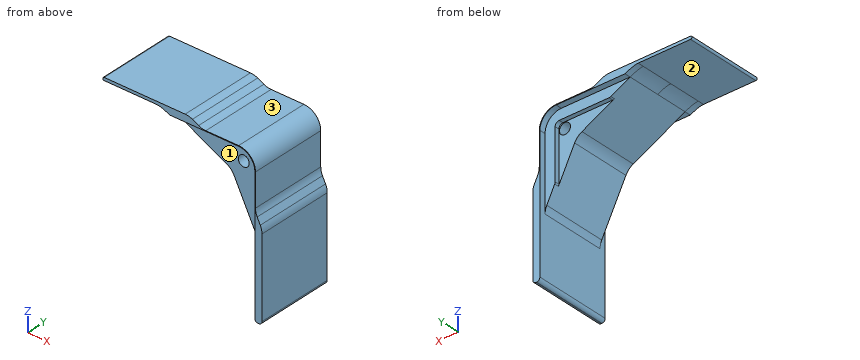
from build123d import *
from build123d.topology import SkipClean

# Parameters (mm, degrees)
SKETCH1_R           = 4.28625
BOSS_EXTRUDE1_DEPTH = 50.8
FILLET8_R           = 12.7
SKETCH2_W           = 42.1132
SKETCH2_H           = 3.302
CUT_EXTRUDE1_DEPTH  = 159.782890609
FILLET3_R           = 2.54
FILLET6_RADIUS      = 1.143
FILLET6_LENGTH      = 50.8
BOSS_EXTRUDE2_DEPTH = 30.1625
CUT_EXTRUDE2_DEPTH  = 163.081683202
FILLET7_R           = 12.7
SKETCH7_W           = 42.968170869
SKETCH7_H           = 42.968170869
CUT_EXTRUDE3_DEPTH  = 3.429
FILLET9_R           = 3.175


with BuildPart() as part:
    # Sketch1 → Boss-Extrude1 (new body)
    with BuildSketch(Plane(origin=(0, 0, 0), x_dir=(1, 0, 0), z_dir=(0, 1, 0))):
        with BuildLine():
            Line((12.7, 53.934971632), (-9.469611004, 9.469611004))
            Line((-9.469611004, 9.469611004), (-53.934971632, -12.7))
            Line((-53.934971632, -12.7), (-106.3752, -12.7))
            Line((-106.3752, -12.7), (-106.3752, -18.288))
            Line((-106.3752, -18.288), (0, -18.288))
            ThreePointArc((0, -18.288), (12.931568814, -12.931568814), (18.288, 0))
            Line((18.288, 0), (18.288, 106.3752))
            Line((18.288, 106.3752), (12.7, 106.3752))
            Line((12.7, 106.3752), (12.7, 53.934971632))
        make_face()
        with Locations(Location((0, 0, 0), (0, 0, 270))):
            Circle(SKETCH1_R, mode=Mode.SUBTRACT)
    extrude(amount=BOSS_EXTRUDE1_DEPTH)

    # Fillet8
    fillet8_edges = [part.edges().sort_by_distance(p)[0] for p in [
        (12.7, 25.4, -53.934971632),
        (-9.469611004, 25.4, -9.469611004),
    ]]
    fillet(fillet8_edges, radius=FILLET8_R)

    # Sketch2 → Cut-Extrude1 (cut, through all)
    with BuildSketch(Plane(origin=(0, 50.8, 0), x_dir=(1, 0, 0), z_dir=(0, 1, 0))):
        with Locations((-85.3186, -14.351)):
            Rectangle(SKETCH2_W, SKETCH2_H)
        with BuildLine():
            Line((-53.934971632, -12.7), (-64.262, -12.7))
            Line((-64.262, -12.7), (-64.262, -16.002))
            add(Edge.make_bspline(
                [(-53.934971632, -12.7), (-60.557759049, -16.002), (-64.262, -16.002)],
                knots=[0, 0, 0, 1, 1, 1], degree=2))
        make_face()
    extrude(amount=-CUT_EXTRUDE1_DEPTH, mode=Mode.SUBTRACT)

    # Fillet3
    fillet3_edges = [part.edges().sort_by_distance(p)[0] for p in [
        (12.7, 25.4, -106.3752),
        (18.288, 25.4, -106.3752),
    ]]
    fillet(fillet3_edges, radius=FILLET3_R)

    # Fillet6: full round fillet: the end face becomes a half cylinder, R = half its width
    fillet6_face = Plane((-106.3752, 25.4, 17.145), x_dir=(0, 1, 0), z_dir=(-1, 0, 0))  # on the end face: x along it, z out of the body
    fillet6_slab = fillet6_face.offset(-FILLET6_RADIUS / 2) * Box(FILLET6_LENGTH, 2 * FILLET6_RADIUS, FILLET6_RADIUS, mode=Mode.PRIVATE)  # the body's end, R deep
    fillet6_round = Plane((-105.2322, 25.4, 17.145), x_dir=(-1, 0, 0), z_dir=(0, 1, 0)) * Cylinder(FILLET6_RADIUS, FILLET6_LENGTH, mode=Mode.PRIVATE)  # its axis R under the face
    add(fillet6_slab - fillet6_round, mode=Mode.SUBTRACT)

    # Sketch3 → Boss-Extrude2 (add, symmetric)
    with SkipClean():  # the faces are left unmerged after this step: merging them gives an invalid solid
        with BuildSketch(Plane(origin=(0, 25.4, 0), x_dir=(1, 0, 0), z_dir=(0, 1, 0))):
            with BuildLine():
                Line((15.748, 106.3752), (15.24, 106.3752))
                ThreePointArc((15.24, 106.3752), (13.443948776, 105.631251224), (12.7, 103.8352))
                Line((12.7, 103.8352), (12.7, 0))
                ThreePointArc((12.7, 0), (8.980256121, -8.980256121), (0, -12.7))
                Line((0, -12.7), (-53.934971632, -12.7))
                add(Edge.make_bspline(
                    [(-53.934971632, -12.7), (-60.557759049, -16.002), (-64.262, -16.002)],
                    knots=[0, 0, 0, 1, 1, 1], degree=2))
                Line((-64.262, -16.002), (-105.2322, -16.002))
                ThreePointArc((-105.2322, -16.002), (-106.3752, -17.145), (-105.2322, -18.288))
                Line((-105.2322, -18.288), (0, -18.288))
                ThreePointArc((0, -18.288), (12.931568814, -12.931568814), (18.288, 0))
                Line((18.288, 0), (18.288, 103.8352))
                ThreePointArc((18.288, 103.8352), (17.544051224, 105.631251224), (15.748, 106.3752))
            make_face()
        extrude(amount=BOSS_EXTRUDE2_DEPTH, both=True)
    add(part.part.scale(1), mode=Mode.REPLACE)  # the faces are merged on a copy

    # Sketch6 → Cut-Extrude2 (cut, through all)
    with BuildSketch(Plane(origin=(0, 55.5625, 0), x_dir=(1, 0, 0), z_dir=(0, 1, 0))):
        with BuildLine():
            Line((-38.862, -18.288), (0, -18.288))
            ThreePointArc((0, -18.288), (12.931568814, -12.931568814), (18.288, 0))
            Line((18.288, 0), (18.288, 38.862))
            Line((18.288, 38.862), (13.208, 28.673096282))
            Line((13.208, 28.673096282), (13.208, 0))
            ThreePointArc((13.208, 0), (9.339466366, -9.339466366), (0, -13.208))
            Line((0, -13.208), (-28.673096282, -13.208))
            Line((-28.673096282, -13.208), (-38.862, -18.288))
        make_face()
    extrude(amount=-CUT_EXTRUDE2_DEPTH, mode=Mode.SUBTRACT)

    # Fillet7
    fillet7_edges = [part.edges().sort_by_distance(p)[0] for p in [
        (13.208, 25.4, -28.673096282),
        (18.288, 25.4, -38.862),
        (-38.862, 25.4, 18.288),
        (-28.673096282, 25.4, 13.208),
    ]]
    fillet(fillet7_edges, radius=FILLET7_R)

    # Sketch7 → Cut-Extrude3 (cut)
    with BuildSketch(Plane(origin=(0, 50.8, 0), x_dir=(1, 0, 0), z_dir=(0, 1, 0))):
        with Locations((-16.658085435, 16.658085435)):
            Rectangle(SKETCH7_W, SKETCH7_H)
    extrude(amount=-CUT_EXTRUDE3_DEPTH, mode=Mode.SUBTRACT)

    # Fillet9
    fillet9_edges = [part.edges().sort_by_distance(p)[0] for p in [
        (4.826, 49.0855, -38.142170869),
        (4.826, 49.0855, 4.826),
        (-38.142170869, 49.0855, 4.826),
    ]]
    fillet(fillet9_edges, radius=FILLET9_R)


solid = part.part
The listing builds one solid part. Answer for the finished solid, in the listing's coordinates (mm). Face numbers are marked on the shaded views. A direction names the side the tool comes from. Give positions to 0.01 mm unless a question says otherwise; leave off trailing zeros. Write each loop counter-clockwise with the first axis right and the second up, starting at its lowest first coordinate (ties: lowest second). Pieces come first, ordered by that corner, then holes. Notation, with made-up numbers: (21, 20.25) -> (33, 20.25) arc R26 ccw to (33, 53.25) -> close; hole circle Ø8 at (77, 24). An arc over 180 degrees is marked (long way). Use a Markdown table: item, result.
(1) Flat-ended cylindrical pins translate along their axes: P1, Ø10, axis at x = -69.5, y = 24.5, coming from the -Z side; P2, Ø6, axis at x = -7, y = 28.5, coming from the -Z side; P3, Ø20.5, axis at x = -9, y = 19, coming from the +Z side. Find the tip coordinate at first contact, or state that the pin passes through.
Return value:
| item | result |
|---|---|
| P1 | z = 16 |
| P2 | z = -20.44 |
| P3 | z = 13.21 |
(2) Section B-B, the plane z = -1.5 is taken. Determine the outline of the cut face in (x, y).
Return value:
| item | result |
|---|---|
| outline | (-25.45, 0) -> (-4.02, 0) -> (-4.02, 47.37) -> (-25.45, 47.37) -> close; (4.02, 0) -> (12.7, 0) -> (12.7, -4.76) -> (13.21, -4.76) -> (13.21, 55.56) -> (12.7, 55.56) -> (12.7, 50.8) -> (4.83, 50.8) -> (4.83, 47.37) -> (4.02, 47.37) -> close |
(3) Section C-C, the plane z = -34 is taken. Determine the outline of the cut face in (x, y), then the cut area to 3 significant figures.
Return value:
| item | result |
|---|---|
| outline | (2.76, 0) -> (12.7, 0) -> (12.7, -4.76) -> (15.86, -4.76) -> (15.86, 55.56) -> (12.7, 55.56) -> (12.7, 50.8) -> (4.83, 50.8) -> (4.83, 47.37) -> (2.76, 47.37) -> close |
| area | 689 mm2 |
(4) Section A-A, the plane x = -2 is taken. Determine the outline of the cut face in (y, z), then the cut area to 3 significant figures.
Return value:
| item | result |
|---|---|
| outline | (-4.76, 12.7) -> (0, 12.7) -> (0, 3.79) -> (47.37, 3.79) -> (47.37, 4.83) -> (50.8, 4.83) -> (50.8, 12.7) -> (55.56, 12.7) -> (55.56, 13.21) -> (-4.76, 13.21) -> close; (0, -24.45) -> (47.37, -24.45) -> (47.37, -3.79) -> (0, -3.79) -> close |
| area | 1,460 mm2 |
(5) For the marked faces 1, 2 and 3, determine the directions among +Z, -Z, +X, -X, +Y, -Y from which every point of the face is accessible in a straight line to the end or side of a thin tool.
Return value:
| item | result |
|---|---|
| face 1 | -Z, -X, -Y |
| face 2 | -Z, -X, +Y, -Y |
| face 3 | +Z, +X, +Y, -Y |
(6) Section D-D, the plane x = -91 is taken. Determine the outline of the cut face in (y, z).
Return value:
| item | result |
|---|---|
| outline | (-4.76, 16) -> (55.56, 16) -> (55.56, 18.29) -> (-4.76, 18.29) -> close |
(7) Find the intervals of material crossed by probe 1 along Z at (x, y) = (-60, 5); probe 2 along X at (y, z) = (8.5, -98.5); probe 3 along Z at (x, y) = (-96.5, 47), in increasing order. Write a range as from..to.
Return value:
| item | result |
|---|---|
| probe 1 | 15.23..18.29 |
| probe 2 | 12.7..18.29 |
| probe 3 | 16..18.29 |
